from build123d import *

# Parameters (mm, degrees)
F1_DEPTH = 10
F2_R     = 7.5
F3_DEPTH = 30


with BuildPart() as f1:
    # F0 (on Top) → F1 (new body)
    with BuildSketch(Plane.XY):
        with BuildLine():
            Line((-2, 9.948416), (-2, 7.228416))
            ThreePointArc((-2, 7.228416), (0, -7.5), (2, 7.228416))
            Line((2, 7.228416), (2, 9.948416))
            Line((2, 9.948416), (-2, 9.948416))
        make_face()
    extrude(amount=F1_DEPTH)

    # F2 (on face) → F3 (join)
    with BuildSketch(Plane.XY.offset(10)):
        Circle(F2_R)
    extrude(amount=F3_DEPTH)


solid = f1.part
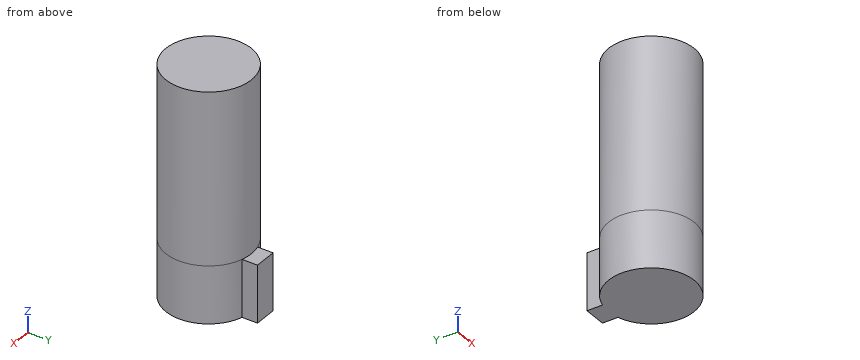
Part model, mm, in its own coordinate system. Coordinates: 2 decimals unless noted, no trailing zeros. Write each loop counter-clockwise with the first axis right and the second up, starting at its lowest first coordinate (ties: lowest second). Pieces come first, ordered by that corner, then holes. Notation, with made-up numbers: (68, 64.25) - (84, 64.25) arc R3 ccw to (84, 68.25) - close; hole circle Ø10 at (88, 40). An arc over 180 degrees is marked (long way). Put each result on its own line as item: value.
1. Probe line 1 along Z through (x, y) = (-1.5, 8.75); line 2 along X through (y, z) = (9, 9.5); line 3 along Y through (x, z) = (3.25, 24). List the from-to ranges inside material, lowest first. Write a range as [from, to].
Final values:
line 1: z = [0, 10]
line 2: x = [-2, 2]
line 3: y = [-6.76, 6.76]
2. Band-saw the part on C-C (y = 2.25). Write the cut outline in (x, z), then the cut area to 3 significant figures.
Final values:
outline: (-7.15, 0) - (7.15, 0) - (7.15, 40) - (-7.15, 40) - close
area: 572 mm²
3. Band-saw the part on A-A (x = 0). Write the cut outline in (y, z), then the cut area to 3 significant figures.
Final values:
outline: (-7.5, 0) - (9.95, 0) - (9.95, 10) - (7.5, 10) - (7.5, 40) - (-7.5, 40) - close
area: 624 mm²
4. Band-saw the part on D-D (z = 7). Write the cut outline in (x, y).
Final values:
outline: (-2, 7.23) arc R7.5 ccw (long way) to (2, 7.23) - (2, 9.95) - (-2, 9.95) - close
5. Flat gauge pins, fed straight in: pin 1 Ø5 at (y, z) = (-4.5, 10) entering from +X; pin 2 Ø1.4 at (x, y) = (0, 9) entering from +Z; pin 3 Ø2 at (y, z) = (8.5, 4) entering from -X. Where does each tip first touch, or does it go through?
Final values:
pin 1: stops at x = 7.23
pin 2: stops at z = 10
pin 3: stops at x = -2
6. Band-saw the part on B-B (z = 36). Write the cut outline in (x, y).
Final values:
outline: circle Ø15 at (0, 0)
